```python
from build123d import *

# Parameters (mm, degrees)
F0_R     = 7.5
F1_DEPTH = 50
F2_R     = 7.5
F3_DEPTH = 30
F3_TAPER = 10
F4_R     = 7.5
F4_R_2   = 2.5
F5_DEPTH = 15


with BuildPart() as f1:
    # F0 (on Top) → F1 (new body)
    with BuildSketch(Plane.XY):
        with Locations((-41.049785912, 39.0788912773)):
            Circle(F0_R)
    extrude(amount=F1_DEPTH)

    # F2 (on face) → F3 (cut)
    with BuildSketch(Plane(origin=(0, 0, 0), x_dir=(1, 0, 0), z_dir=(0, 0, -1))):
        with Locations((-41.049785912, -39.0788912773)):
            Circle(F2_R)
    extrude(amount=-F3_DEPTH, taper=F3_TAPER, mode=Mode.SUBTRACT)

    # F4 (on face) → F5 (cut)
    with BuildSketch(Plane.XY.offset(50)):
        with Locations((-41.049785912, 39.0788912773)):
            Circle(F4_R)
        with Locations((-41.049785912, 39.0788912773)):
            Circle(F4_R_2, mode=Mode.SUBTRACT)
    extrude(amount=-F5_DEPTH, mode=Mode.SUBTRACT)


solid = f1.part
```
Read the model definition and answer for the solid it produces. Units are mm, in the model's axes. A direction names the side the tool comes from. Round coordinates to 2 decimals unless told otherwise and drop trailing zeros. Loops run counter-clockwise (first coordinate to the right, second up) from the corner with the lowest first, then second, coordinate; pieces in that order, holes last. Notation, with made-up numbers: (43.25, 52) -> (102.25, 52) arc R32 cw to (102.25, 88) -> close; hole circle Ø2 at (-10.75, 69). An arc over 180 degrees is marked (long way). One line per item, written item: value.
1) A cutting plane is placed at C-C (z = 10). Determine the outline of the cut face in (x, y).
Answer list:
outline: circle Ø15 at (-41.05, 39.08); hole circle Ø11.47 at (-41.05, 39.08)
2) A cutting plane is placed at B-B (z = 44). Determine the outline of the cut face in (x, y), and give its area (3 significant figures).
Answer list:
outline: circle Ø5 at (-41.05, 39.08)
area: 19.6 mm²
3) Flat-ended cylindrical pins translate along their axes: P1, Ø3, axis at x = -40.5, y = 43.5, coming from the +Z side; P2, Ø1, axis at x = -39, z = 11.5, coming from the +Y side; P3, Ø3, axis at x = -46.5, z = 32.5, coming from the -Y side. Find the tip coordinate at first contact, or state that the pin passes through.
Answer list:
P1: stops at z = 35
P2: stops at y = 46.42
P3: stops at y = 32.7
4) A cutting plane is placed at D-D (z = 33.5). Determine the outline of the cut face in (x, y).
Answer list:
outline: circle Ø15 at (-41.05, 39.08)
5) A cutting plane is placed at A-A (z = 17). Determine the outline of the cut face in (x, y), and give its area (3 significant figures).
Answer list:
outline: circle Ø15 at (-41.05, 39.08); hole circle Ø9 at (-41.05, 39.08)
area: 113 mm²
6) Consider L1, parallel to Y at x = -45.5, z = 14; L2, parallel to X at y = 39.5, z = 9.5; L3, parallel to X at y = 37, z = 3. Determine where each line is inside the solid, lowest interval first. Write a range as [from, to].
Answer list:
L1: y = [33.04, 36.73], [41.43, 45.12]
L2: x = [-48.54, -46.86], [-35.24, -33.56]
L3: x = [-48.26, -47.7], [-34.4, -33.84]
7) For faces 5 (the face through (-43, 41, 35)), 6 (the face through (-48.543, 39.409, 17.255)), determine the directions among +Z, -Z, +X, -X, +Y, -Y from which every point of the face is accessible in a straight line to the end or side of a thin tool.
Answer list:
face 5: +Z
face 6: +Z, -Z
8) The mould has two halves that part along X. Classify faces 1 (the face through (-41, 39, 50)), 2 (the face through (-42.89, 40.77, 42.6)), 3 (the face through (-41, 39, 30)), 4 (the face through (-38.827, 43.353, 15.21)): pulls with the +X half, pulls with the -X half, needs draft (parallel to the pull), parting line crosses it, or undercut.
Answer list:
face 1: needs draft
face 2: parting line crosses it
face 3: undercut
face 4: undercut
